Job drawing, mm, ordinate dimensions from the low corner. One solid piece. Give positions to 0.01 mm unless a question says otherwise; leave off trailing zeros. Write each loop counter-clockwise with the first axis right and the second up, starting at its lowest first coordinate (ties: lowest second). Pieces come first, ordered by that corner, then holes. Notation, with made-up numbers: (7.25, 41.5) -> (65.25, 41.5) arc R19 ccw to (65.25, 45.5) -> close; hole circle Ø3 at (-12, 68). An arc over 180 degrees is marked (long way). Put each result on its own line as item: value. Start each with the question number.
Item 1: Slice it at C-C, the plane x = 4. List the corners of the cut face in (y, z).
Item 2: Drill centre lines: line 1 along X through (y, z) = (4, 8.75); line 2 along Z through (x, y) = (7.75, 3); line 3 along Y through (x, z) = (5, 17.75). Where is each one in solid material? Low to high.
Item 3: Flat gauge pins, fed straight in: pin 1 Ø4 at (x, z) = (2, 11) entering from +Y; pin 2 Ø1 at (y, z) = (2.5, 16.5) entering from +X; pin 3 Ø1.7 at (y, z) = (5, 2.5) entering from -X. Where does each tip first touch, or does it go through?
Item 4: Slice it at B-B, the plane y = 4. List the corners of the cut face in (x, z), plus the area to 3 significant figures.
Item 5: Slice it at A-A, the plane x = 2.5. List the corners of the cut face in (y, z), plus the area to 3 significant figures.
Item 6: Two-plate mould, pull along Z, no slides. Class the marked faces 1, 2, 3 and 4: pulls with the +Z half, pulls with the -Z half, needs draft (parallel to the pull), parting line crosses it, or undercut.
Item 7: Slice it at D-D, the plane z = 11.75. List the corners of the cut face in (x, y).
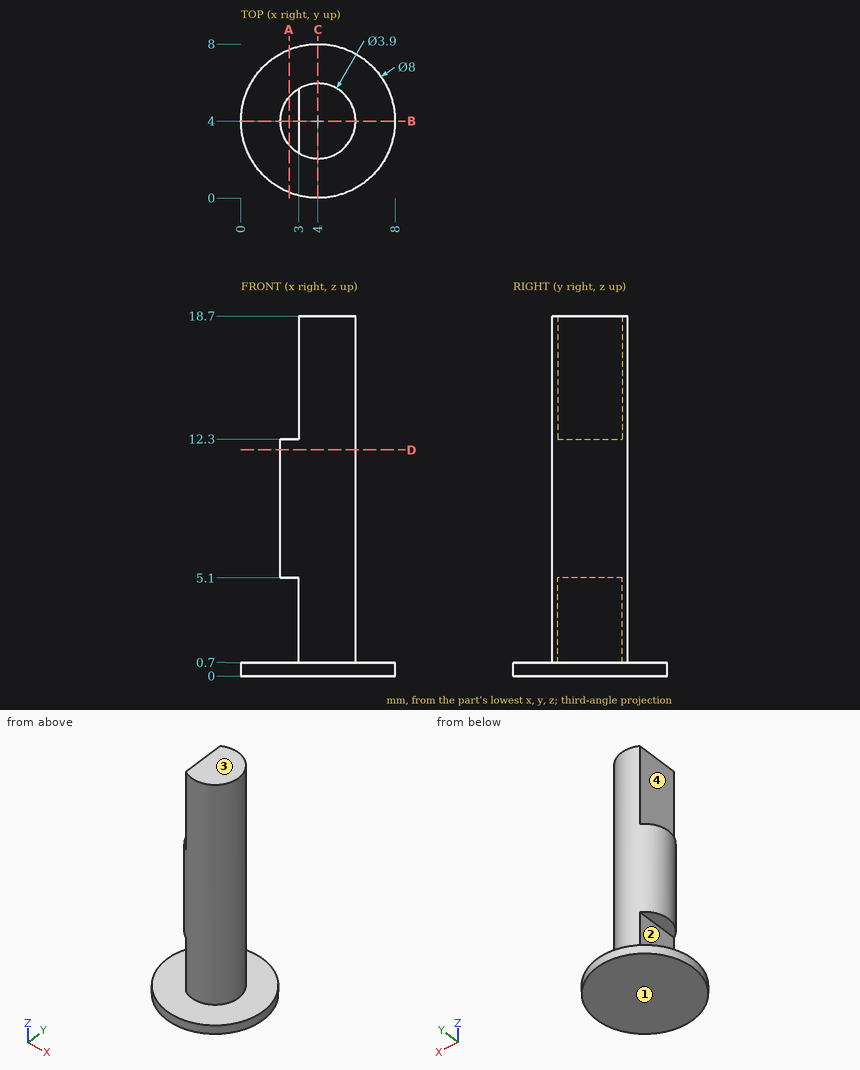
Values follow:
1. outline: (0, 0) -> (8, 0) -> (8, 0.7) -> (5.95, 0.7) -> (5.95, 18.7) -> (2.05, 18.7) -> (2.05, 0.7) -> (0, 0.7) -> close
2. line 1: 2.05 to 5.95
2. line 2: 0 to 0.7
2. line 3: 2.33 to 5.67
3. pin 1: y = 5.95
3. pin 2: x = 5.67
3. pin 3: x = 3
4. outline: (0, 0) -> (8, 0) -> (8, 0.7) -> (5.95, 0.7) -> (5.95, 18.7) -> (3, 18.7) -> (3, 12.3) -> (2.05, 12.3) -> (2.05, 5.1) -> (3, 5.1) -> (3, 0.7) -> (0, 0.7) -> close
4. area: 65.5 mm2
5. outline: (0.29, 0) -> (7.71, 0) -> (7.71, 0.7) -> (0.29, 0.7) -> close; (2.75, 5.1) -> (5.25, 5.1) -> (5.25, 12.3) -> (2.75, 12.3) -> close
5. area: 23.1 mm2
6. face 1: pulls with the -Z half
6. face 2: undercut
6. face 3: pulls with the +Z half
6. face 4: needs draft
7. outline: circle Ø3.9 at (4, 4)
